```python
from build123d import *

# Parameters (mm, degrees)
SKETCH4_R           = 31.75
SKETCH4_R_2         = 20.2
BOSS_EXTRUDE1_DEPTH = 3
FILLET1_R           = 2
FILLET2_R           = 2
BOSS_EXTRUDE2_DEPTH = 1
CIRPATTERN1_COUNT   = 4
CUT_EXTRUDE1_DEPTH  = 6
CUT_EXTRUDE2_DEPTH  = 6


with BuildPart() as part:
    # Sketch3 → Revolve1 (revolve)
    with BuildSketch(Plane.XY):
        Polygon((-22.571572875, 0), (-25.4, 0), (-22.2, 3.2), (-22.2, 25.4), (-20.2, 25.4), (-20.2, 2.371572875), align=None)
    revolve(axis=Axis((0, 25.4, 0), (0, -1, 0)))

    # Sketch4 → Boss-Extrude1 (add)
    with BuildSketch(Plane.XZ):
        Circle(SKETCH4_R)
        Circle(SKETCH4_R_2, mode=Mode.SUBTRACT)
    extrude(amount=BOSS_EXTRUDE1_DEPTH)

    # Fillet1
    fillet1_edges = [part.edges().sort_by_distance(p)[0] for p in [
        (25.4, 0, 0),
    ]]
    fillet(fillet1_edges, radius=FILLET1_R)

    # Fillet2
    fillet2_edges = [part.edges().sort_by_distance(p)[0] for p in [
        (22.2, 3.2, 0),
    ]]
    fillet(fillet2_edges, radius=FILLET2_R)

    # Sketch5 → Boss-Extrude2 (add, symmetric)
    with BuildSketch(Plane.XY):
        Polygon((20.2, 0), (23.444013634, 0), (23.444013634, 1.439043573), (20.2, 4.645223745), align=None)
    boss_extrude2 = extrude(amount=BOSS_EXTRUDE2_DEPTH, both=True)

    # CirPattern1: Boss-Extrude2 ×4 about axis
    cirpattern1_axis = Axis((0, 0, 0), (0, 1, 0))
    for i in range(1, CIRPATTERN1_COUNT):
        add(boss_extrude2.rotate(cirpattern1_axis, i * 360 / CIRPATTERN1_COUNT))

    # Sketch6 → Cut-Extrude1 (cut)
    with BuildSketch(Plane(origin=(0, 25.4, 0), x_dir=(1, 0, 0), z_dir=(0, 1, 0))):
        with BuildLine():
            Line((0, 20), (-13.834891336, 20))
            ThreePointArc((-13.834891336, 20), (0, 24.318803801), (13.834891336, 20))
            Line((13.834891336, 20), (0, 20))
        make_face()
    extrude(amount=-CUT_EXTRUDE1_DEPTH, mode=Mode.SUBTRACT)

    # Sketch7 → Cut-Extrude2 (cut)
    with BuildSketch(Plane(origin=(0, 25.4, 0), x_dir=(1, 0, 0), z_dir=(0, 1, 0))):
        Polygon((-9.635351576, 20), (2.835489376, 20), (9.635351576, 20), (7.753188698, 16.093213904), (-7.753188698, 16.093213904), align=None)
    extrude(amount=-CUT_EXTRUDE2_DEPTH, mode=Mode.SUBTRACT)


solid = part.part
```
The listing builds one solid part. Answer for the finished solid, in the listing's coordinates (mm). A direction names the side the tool comes from. Round coordinates to 2 decimals unless told otherwise and drop trailing zeros. Loops run counter-clockwise (first coordinate to the right, second up) from the corner with the lowest first, then second, coordinate; pieces in that order, holes last. Notation, with made-up numbers: (81, 19) - (132, 19) arc R32 cw to (132, 58) - close; hole circle Ø9 at (-24.75, 12). An arc over 180 degrees is marked (long way). Use one line per item in the form item = value. Start each with the question number.
1. Given pin 1 Ø1.6 at (y, z) = (2, -0.5) entering from -X (3 decimals); pin 2 Ø1.6 at (x, y) = (0, 1) entering from +Z; pin 3 Ø4.5 at (x, z) = (-2.5, -19.5) entering from +Y; pin 4 Ø18 at (x, z) = (-14.5, 10.5) entering from +Y, each flat-ended and moving along its own axis, determine where each tip first touches the part or whether it passes through.
2. The part is cut by section A-A on y = 7.25. Determine the outline of the cut face in (x, z), then the cut area to 3 significant figures.
3. A tool of negligible diameter and unlimited length cuts with its end or side. For faces 3 (the face through (21, 1, -1)), 4 (the face through (0, 19.4, -21)), from which of +Z, -Z, +X, -X, +Y, -Y can it reach the whole face along a straight path? Write none if from no direction.
4. Consider line 1 (Z direction, x = 0, y = 12.25); line 2 (Z direction, x = 0, y = -1.25). Determine where each line is inside the solid, lowest interval first. Write a range as [from, to].
5. The part is cut by section B-B on y = 23. Determine the outline of the cut face in (x, z), then the cut area to 3 significant figures.
6. For a pull along X with two mould halves and no side action, classify faces 1 (the face through (15, 0, -15)), 2 (the face through (0, -3, -21)) as pulls with the +X half, pulls with the -X half, needs draft (parallel to the pull), parting line crosses it, or undercut.
Geometry check:
q1.pin_1 = -24.195
q1.pin_2 = 25.36
q1.pin_3 = 19.4
q1.pin_4 = 25.4
q2.outline = circle Ø44.4 at (0, 0); hole circle Ø40.4 at (0, 0)
q2.area = 266 mm^2
q3.face_3 = none
q3.face_4 = -Z, +Y
q4.line_1 = [-22.2, -20.2], [20.2, 22.2]
q4.line_2 = [-31.75, -20.2], [20.2, 31.75]
q5.outline = (-9.64, -20) - (-8.77, -18.2) arc R20.2 cw (long way) to (8.77, -18.2) - (9.64, -20) arc R22.2 ccw (long way) to start
q5.area = 228 mm^2
q6.face_1 = undercut
q6.face_2 = needs draft
